Geometry check sheet. Reference: drawing and pictorial views, mm from the part's lowest x, y, z. A direction names the side the tool comes from. Give positions to 0.01 mm unless a question says otherwise; leave off trailing zeros. Loops run counter-clockwise (first coordinate to the right, second up) from the corner with the lowest first, then second, coordinate; pieces in that order, holes last. Notation, with made-up numbers: (74.5, 14) - (130.5, 14) arc R5 ccw to (130.5, 23) - close; hole circle Ø1 at (10, -10.5). An arc over 180 degrees is marked (long way). Use CSV: the item, a comma, the result in double quotes.
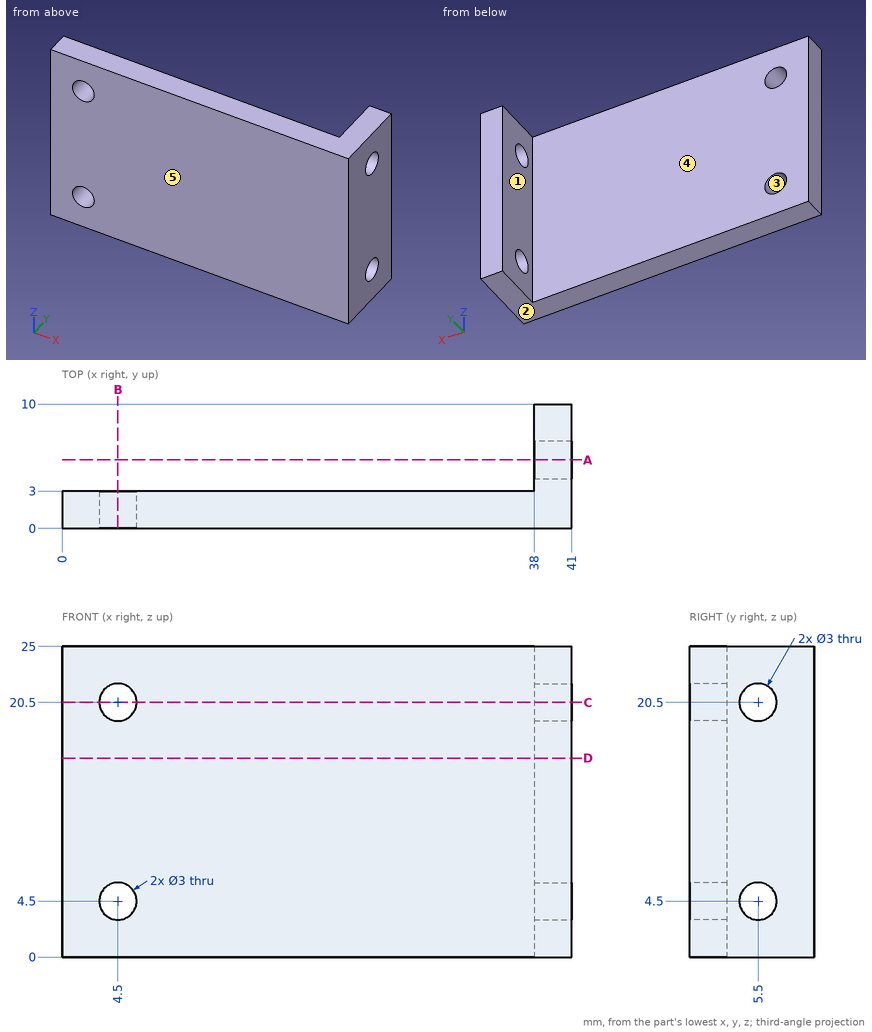
1. Sectioned sample at C-C, the plane z = 20.5. Record the boundary of the cut face in (x, y), and give its area (3 significant figures).
Completed:
outline,"(0, 0) - (3, 0) - (3, 3) - (0, 3) - close; (6, 0) - (41, 0) - (41, 4) - (38, 4) - (38, 3) - (6, 3) - close; (38, 7) - (41, 7) - (41, 10) - (38, 10) - close"
area,"126 mm²"
2. Sectioned sample at D-D, the plane z = 16. Record the boundary of the cut face in (x, y), and give its area (3 significant figures).
Completed:
outline,"(0, 0) - (41, 0) - (41, 10) - (38, 10) - (38, 3) - (0, 3) - close"
area,"144 mm²"
3. Go/stop test with flat-tipped pins: pin 1 Ø3.5 at (y, z) = (7, 14.5) entering from -X; pin 2 Ø1 at (x, z) = (23, 17.5) entering from +Y. Record where each tip stops, or that it passes through.
Completed:
pin 1,"stops at x = 38"
pin 2,"stops at y = 3"
4. Release check for a two-part mould opening along X. For the marked faces 1, 2 and 3 record: released by +X, released by -X, zero draft, split by the parting line, or undercut.
Completed:
face 1,"released by -X"
face 2,"zero draft"
face 3,"undercut"
5. Scan lines: line 1 along Z through (x, y) = (4.5, 0.75); line 2 along Y through (x, z) = (8, 12); line 3 along X through (y, z) = (8.5, 17.5). Record each from-to range of solid material in increasing order.
Completed:
line 1,"z = 0 to 3, 6 to 19, 22 to 25"
line 2,"y = 0 to 3"
line 3,"x = 38 to 41"
6. Set-up check for the marked faces 4 and 5: record each of +Z, -Z, +X, -X, +Y, -Y from which the full face is reachable in a straight line by a thin tool's end or side.
Completed:
face 4,"+Z, -Z, -X, +Y"
face 5,"+Z, -Z, +X, -X, -Y"
7. Sectioned sample at A-A, the plane y = 5.5. Record the boundary of the cut face in (x, z).
Completed:
outline,"(38, 0) - (41, 0) - (41, 3) - (38, 3) - close; (38, 6) - (41, 6) - (41, 19) - (38, 19) - close; (38, 22) - (41, 22) - (41, 25) - (38, 25) - close"
8. Sectioned sample at B-B, the plane x = 4.5. Record the boundary of the cut face in (y, z), and give its area (3 significant figures).
Completed:
outline,"(0, 0) - (3, 0) - (3, 3) - (0, 3) - close; (0, 6) - (3, 6) - (3, 19) - (0, 19) - close; (0, 22) - (3, 22) - (3, 25) - (0, 25) - close"
area,"57.0 mm²"
